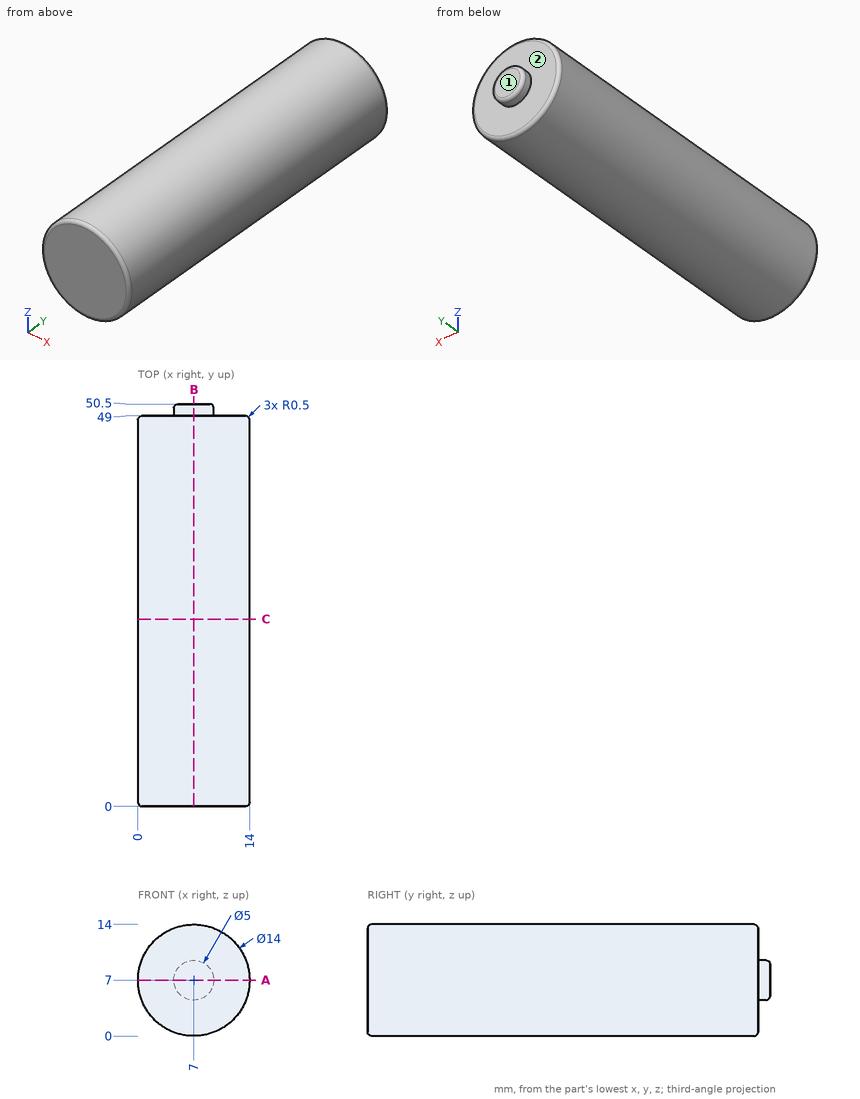
Here's the drawing with two shaded views (mm, measured from the low corner). I have some questions. A direction names the side the tool comes from. Give positions to 0.01 mm unless a question says otherwise; leave off trailing zeros. Order: outer loops, then holes, each group sorted by start corner. A loop starts at its lowest first (then second) coordinate and runs counter-clockwise, first axis right, second up. Notation, with made-up numbers: (48, 89.25) - (107, 89.25) arc R22 ccw to (107, 128.25) - close; hole circle Ø11 at (-15.5, 16). An arc over 180 degrees is marked (long way). Use a Markdown table: item, result. Add a question column.
Q1. If we section it at C-C on y = 23.5: Write out the boundary of the cut face in (x, z), plus the area to 3 significant figures.
Q2. If we section it at A-A on z = 7: Write out the boundary of the cut face in (x, y).
Q3. If we section it at B-B on x = 7: Write out the boundary of the cut face in (y, z), plus the area to 3 significant figures.
Q4. Please list where these lines run through material, in increasing order: line 1 along Y through (x, z) = (3.25, 2); line 2 along X through (y, z) = (7.5, 0.75); line 3 along Z through (x, y) = (1.25, 43).
Q5. I'm going to push flat-ended pins straight in: pin 1 (3 mm diameter, centred on y = 9.5, z = 4.5, fed in from +X); pin 2 (4 mm diameter, centred on y = 30, z = 11.5, fed in from -X). Where does each tip first touch, or does it pass through?
Q6. On a 3-axis mill with a long thin cutter (end or side, diameter ignored), from which of +Z, -Z, +X, -X, +Y, -Y can I reach the whole of each face in a straight line? I mean the marked faces 1 and 2. Say none if no direction works.
Answers follow:
| question | item | result |
|---|---|---|
| 1 | outline | circle Ø14 at (7, 7) |
| 1 | area | 154 mm^2 |
| 2 | outline | (0, 0.5) arc R0.5 ccw to (0.5, 0) - (13.5, 0) arc R0.5 ccw to (14, 0.5) - (14, 48.5) arc R0.5 ccw to (13.5, 49) - (9.5, 49) - (9.5, 50) arc R0.5 ccw to (9, 50.5) - (5, 50.5) arc R0.5 ccw to (4.5, 50) - (4.5, 49) - (0.5, 49) arc R0.5 ccw to (0, 48.5) - close |
| 3 | outline | (0, 0.5) arc R0.5 ccw to (0.5, 0) - (48.5, 0) arc R0.5 ccw to (49, 0.5) - (49, 4.5) - (50, 4.5) arc R0.5 ccw to (50.5, 5) - (50.5, 9) arc R0.5 ccw to (50, 9.5) - (49, 9.5) - (49, 13.5) arc R0.5 ccw to (48.5, 14) - (0.5, 14) arc R0.5 ccw to (0, 13.5) - close |
| 3 | area | 693 mm^2 |
| 4 | line 1 | y = 0 to 49 |
| 4 | line 2 | x = 3.85 to 10.15 |
| 4 | line 3 | z = 3.01 to 10.99 |
| 5 | pin 1 | stops at x = 13.93 |
| 5 | pin 2 | stops at x = 0.46 |
| 6 | face 1 | +Z, -Z, +X, -X, +Y |
| 6 | face 2 | +Y |
